from build123d import *

# Parameters (mm, degrees)
SKETCH_R      = 65
SKETCH_R_2    = 20
SKETCH_R_3    = 2.25
EXTRUDE_DEPTH = 4


with BuildPart() as part:
    # Sketch → Extrude (new body)
    with BuildSketch(Plane.XY):
        Circle(SKETCH_R)
        Circle(SKETCH_R_2, mode=Mode.SUBTRACT)
        with Locations((-24.041631, 24.041631)):
            Circle(SKETCH_R_3, mode=Mode.SUBTRACT)
        with Locations((0, 34)):
            Circle(SKETCH_R_3, mode=Mode.SUBTRACT)
        with Locations((34, 0)):
            Circle(SKETCH_R_3, mode=Mode.SUBTRACT)
        with Locations((0, -34)):
            Circle(SKETCH_R_3, mode=Mode.SUBTRACT)
        with Locations((-24.041631, -24.041631)):
            Circle(SKETCH_R_3, mode=Mode.SUBTRACT)
        with Locations((-34, 0)):
            Circle(SKETCH_R_3, mode=Mode.SUBTRACT)
        with Locations((24.041631, -24.041631)):
            Circle(SKETCH_R_3, mode=Mode.SUBTRACT)
        with Locations((24.041631, 24.041631)):
            Circle(SKETCH_R_3, mode=Mode.SUBTRACT)
        with Locations((41.012193, 41.012193)):
            Circle(SKETCH_R_3, mode=Mode.SUBTRACT)
        with Locations((-58, 0)):
            Circle(SKETCH_R_3, mode=Mode.SUBTRACT)
        with Locations((0, -58)):
            Circle(SKETCH_R_3, mode=Mode.SUBTRACT)
        with Locations((-41.012193, -41.012193)):
            Circle(SKETCH_R_3, mode=Mode.SUBTRACT)
        with Locations((-41.012193, 41.012193)):
            Circle(SKETCH_R_3, mode=Mode.SUBTRACT)
        with Locations((41.012193, -41.012193)):
            Circle(SKETCH_R_3, mode=Mode.SUBTRACT)
        with Locations((0, 58)):
            Circle(SKETCH_R_3, mode=Mode.SUBTRACT)
        with Locations((58, 0)):
            Circle(SKETCH_R_3, mode=Mode.SUBTRACT)
    extrude(amount=EXTRUDE_DEPTH)


solid = part.part
For this review, take the finished solid that the model builds, in its own axes (mm). Round coordinates to 2 decimals unless told otherwise and drop trailing zeros. Order: outer loops, then holes, each group sorted by start corner. A loop starts at its lowest first (then second) coordinate and runs counter-clockwise, first axis right, second up. Notation, with made-up numbers: (63, -35.5) -> (83, -35.5) arc R20 ccw to (83, -26.5) -> close; hole circle Ø5 at (-2.5, -13.75). An arc over 180 degrees is marked (long way). Write item = value, one per line. Start each with the question number.
1) Take a section at A-A on x = 0. State the section outline as (y, z) points, plus the area to 3 significant figures.
2) Take a section at D-D on x = -34. State the section outline as (y, z) points, plus the area to 3 significant figures.
3) Take a section at C-C on z = 1.9. Count the separate pieces of the cut face and the enclosed holes in it, plus the area to 3 significant figures.
4) The part is to be moulded in two halves that separate along Y. For faces 1 (the face through (14, 15, 0)), 2 (the face through (62, 19.52, 1.97)), 3 (the face through (-25.7, -22.52, 1.97)), say which applies: +Y half, -Y half, draft (parallel to the pull), parting line (faces both ways), or undercut.
5) Take a section at B-B on y = -13. State the section outline as (x, z) points.
6) To check wall thickness, follow line 1 (Y direction, x = 0, z = 2.8); line 2 (X direction, y = -24.5, z = 1.5); line 3 (Y direction, x = 43, z = 2.3). State the ranges of each line that lie inside material, in increasing order. Write a range as from..to.
7) Insertion check: pin 1 (2 mm diameter, centred on x = -40, z = 3.5, fed in from +Y); pin 2 (1.5 mm diameter, centred on x = 41.5, z = 0.5, fed in from +Y). Each pin has a flat end and moves straight along its axis. Give the tip position at first contact, or say it passes through.
Verdict:
q1.outline = (-65, 0) -> (-60.25, 0) -> (-60.25, 4) -> (-65, 4) -> close; (-55.75, 0) -> (-36.25, 0) -> (-36.25, 4) -> (-55.75, 4) -> close; (-31.75, 0) -> (-20, 0) -> (-20, 4) -> (-31.75, 4) -> close; (20, 0) -> (31.75, 0) -> (31.75, 4) -> (20, 4) -> close; (36.25, 0) -> (55.75, 0) -> (55.75, 4) -> (36.25, 4) -> close; (60.25, 0) -> (65, 0) -> (65, 4) -> (60.25, 4) -> close
q1.area = 288 mm2
q2.outline = (-55.4, 0) -> (-2.25, 0) -> (-2.25, 4) -> (-55.4, 4) -> close; (2.25, 0) -> (55.4, 0) -> (55.4, 4) -> (2.25, 4) -> close
q2.area = 425 mm2
q3.separate_pieces = 1
q3.enclosed_holes = 17
q3.area = 11,800 mm2
q4.face_1 = draft
q4.face_2 = parting line
q4.face_3 = undercut
q5.outline = (-63.69, 0) -> (-15.2, 0) -> (-15.2, 4) -> (-63.69, 4) -> close; (15.2, 0) -> (63.69, 0) -> (63.69, 4) -> (15.2, 4) -> close
q6.line_1 = -65..-60.25, -55.75..-36.25, -31.75..-20, 20..31.75, 36.25..55.75, 60.25..65
q6.line_2 = -60.21..-26.24, -21.84..21.84, 26.24..60.21
q6.line_3 = -48.74..-42.07, -39.96..39.96, 42.07..48.74
q7.pin_1 = 52
q7.pin_2 = 50.64
